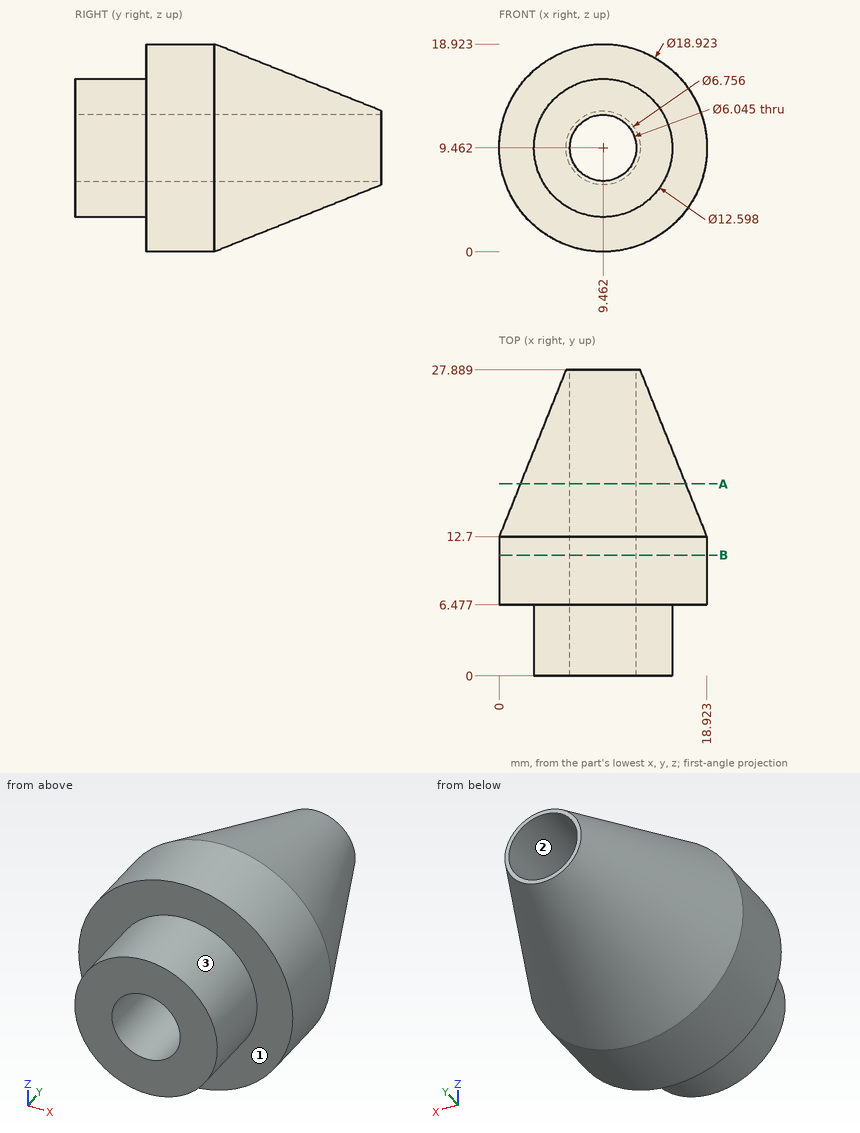
Here's the drawing with two shaded views (mm, measured from the low corner). I have some questions. Give positions to 0.01 mm unless a question says otherwise; leave off trailing zeros. Loops run counter-clockwise (first coordinate to the right, second up) from the corner with the lowest first, then second, coordinate; pieces in that order, holes last. Notation, with made-up numbers: (77, 48.5) - (112, 48.5) arc R14 ccw to (112, 57.5) - close; hole circle Ø11 at (35.5, 72). An arc over 180 degrees is marked (long way). One line per item, written item: value.
(1) I'm going to push flat-ended pins straight in: pin 1 (3 mm diameter, centred on x = 14, y = 10.5, fed in from +Z); pin 2 (6 mm diameter, centred on x = 2, z = 12, fed in from +Y) (1 decimal); pin 3 (6 mm diameter, centred on x = 2.5, y = 15, fed in from +Z); pin 4 (5 mm diameter, centred on x = 9.46, z = 9.46, fed in from -Y). Where does each tip first touch, or does it pass through?
Verdict:
pin 1: z = 18.42
pin 2: y = 24.1
pin 3: z = 17.52
pin 4: through
(2) If we section it at A-A, the plane y = 17.5: List the corners of the cut face in (x, z) for me (1 decimal), plus the area to 3 significant figures.
Verdict:
outline: circle Ø15.1 at (9.5, 9.5); hole circle Ø6 at (9.5, 9.5)
area: 150 mm^2
(3) If we mould it in two halves opening along X, with no side actions, what happens to the marked faces 1, 2 and 3? For each: released by +X, released by -X, zero draft, split by the parting line, or undercut.
Verdict:
face 1: zero draft
face 2: undercut
face 3: split by the parting line
(4) If we section it at B-B, the plane y = 11: List the corners of the cut face in (x, z) for me (1 decimal).
Verdict:
outline: circle Ø18.9 at (9.5, 9.5); hole circle Ø6 at (9.5, 9.5)
(5) I need wall thicknesses on line 1 along Z through (x, y) = (10, 1.25) (1 decimal); line 2 along Z through (x, y) = (7.5, 17.5); line 3 along Z through (x, y) = (5, 12.5) (1 decimal). Which ranges of each line are inside material? Lowest first, please.
Verdict:
line 1: 3.2 to 6.5, 12.4 to 15.7
line 2: 2.18 to 7.16, 11.76 to 16.74
line 3: 1.1 to 17.8
